Input: part model. Units: mm. Frame: model coordinates. A direction names the side the tool comes from. Coordinates: 2 decimals unless noted, no trailing zeros. Loops run counter-clockwise (first coordinate to the right, second up) from the corner with the lowest first, then second, coordinate; pieces in that order, holes last.
(1) Section A-A, the plane x = -22. Return loops of the section in (y, z).
(2) Section B-B, the plane y = 3. Return loops of the section in (x, z).
(3) Section C-C, the plane z = -48. Return loops of the section in (x, y).
(4) Section D-D, the plane z = 0. Return loops of the section in (x, y), then the cut area to 3 significant figures.
(5) Set-up query: faces 5 (the face through (-20, 24, -13)), 6 (the face through (6, 17, -1)), 7 (the face through (0, 15, -18)), 8 (the face through (17.44, 35.07, -33.96)), 9 (the face through (-13, 24, -8)). Return all of +Z, -Z, +X, -X, +Y, -Y with unobstructed straight access to the full face (end or side cutting, diameter ignored); none if empty.
(6) Mould query, pull axis X, two halves, no side actions, for faces 1 (the face through (1, 0, 0)), 2 (the face through (46, 4, 0)), 3 (the face through (35.932, 3.944, -1.041)), 4 (the face through (-6, 17, -1)). Classes: released by +X, released by -X, zero draft, split by the parting line, or undercut.
(7) Line query: L1, parallel to X at y = 6, z = 0; L2, parallel to Z at x = -15, y = 29.5; L3, parallel to Y at x = 5.5, z = -34. Output: solid intervals per line, ascending.
(8) Contact query for flat-ended pins moving along their axis: P1, Ø21, axis at x = -28, z = 0, coming from the +Y side; P2, Ø1, axis at x = -10.5, z = -39, coming from the -Y side; P3, Ø18, axis at x = 21, z = -7, coming from the +Y side. Output: stop coordinate, or through.
```python
from build123d import *

# Parameters (mm, degrees)
SKETCH2_R                = 8
BOSS_EXTRUDE1_DEPTH      = 8
SKETCH4_W                = 40
SKETCH4_H                = 10
BOSS_EXTRUDE2_DEPTH      = 32
BOSS_EXTRUDE3_DEPTH      = 6
BOSS_EXTRUDE3_DEPTH_BACK = 6
SKETCH7_R                = 10
BOSS_EXTRUDE4_DEPTH      = 10
BOSS_EXTRUDE5_START      = 10
SKETCH8_R                = 15
SKETCH8_R_2              = 10
BOSS_EXTRUDE5_DEPTH      = 10


with BuildPart() as part:
    # Sketch2 → Boss-Extrude1 (new body)
    with BuildSketch(Plane(origin=(0, 0, 0), x_dir=(1, 0, 0), z_dir=(0, 1, 0))):
        with BuildLine():
            Line((-28, 18), (28, 18))
            ThreePointArc((28, 18), (46, 0), (28, -18))
            Line((28, -18), (-28, -18))
            ThreePointArc((-28, -18), (-46, 0), (-28, 18))
        make_face()
        with Locations(Location((-28, 0, 0), (0, 0, 270))):
            Circle(SKETCH2_R, mode=Mode.SUBTRACT)
        with Locations(Location((28, 0, 0), (0, 0, 270))):
            Circle(SKETCH2_R, mode=Mode.SUBTRACT)
    extrude(amount=BOSS_EXTRUDE1_DEPTH)

    # Sketch4 → Boss-Extrude2 (add)
    with BuildSketch(Plane(origin=(0, 8, 0), x_dir=(1, 0, 0), z_dir=(0, 1, 0))):
        with Locations((0, 13)):
            Rectangle(SKETCH4_W, SKETCH4_H)
    extrude(amount=BOSS_EXTRUDE2_DEPTH)

    # Sketch5 → Boss-Extrude3 (add, two sides: drawn at the far end of the back side and taken through both)
    with BuildSketch(Plane(origin=(0, 0, 0), x_dir=(0, 0, -1), z_dir=(1, 0, 0)).offset(-BOSS_EXTRUDE3_DEPTH_BACK)):
        Polygon((8, 40), (8, 8), (-18, 8), align=None)
    extrude(amount=BOSS_EXTRUDE3_DEPTH + BOSS_EXTRUDE3_DEPTH_BACK)

    # Sketch7 → Boss-Extrude4 (add)
    with BuildSketch(Plane(origin=(0, 40, 0), x_dir=(1, 0, 0), z_dir=(0, 1, 0))):
        with BuildLine():
            Line((20, 18), (14.810951292, 50.373967528))
            ThreePointArc((14.810951292, 50.373967528), (0, 63), (-14.810951292, 50.373967528))
            Line((-14.810951292, 50.373967528), (-20, 18))
            Line((-20, 18), (20, 18))
        make_face()
        with Locations(Location((0, 48, 0), (0, 0, 270))):
            Circle(SKETCH7_R, mode=Mode.SUBTRACT)
    extrude(amount=-BOSS_EXTRUDE4_DEPTH)

    # Sketch8 → Boss-Extrude5 (add)
    with BuildSketch(Plane(origin=(0, 40, 0), x_dir=(1, 0, 0), z_dir=(0, 1, 0)).offset(BOSS_EXTRUDE5_START)):
        with Locations(Location((0, 48, 0), (0, 0, 270))):
            Circle(SKETCH8_R)
        with Locations(Location((0, 48, 0), (0, 0, 270))):
            Circle(SKETCH8_R_2, mode=Mode.SUBTRACT)
    extrude(amount=-BOSS_EXTRUDE5_DEPTH)


solid = part.part
```
Report:
1. outline: (0, -18) - (8, -18) - (8, -5.29) - (0, -5.29) - close; (0, 5.29) - (8, 5.29) - (8, 18) - (0, 18) - close
2. outline: (-28, -18) - (28, -18) arc R18 ccw to (28, 18) - (-28, 18) arc R18 ccw to start; hole circle Ø16 at (-28, 0); hole circle Ø16 at (28, 0)
3. outline: (-15.19, 30) - (-10, 30) - (-10, 50) - (-15, 50) - (-15, 40) - (-15.19, 40) - close; (10, 30) - (15.19, 30) - (15.19, 40) - (15, 40) - (15, 50) - (10, 50) - close
4. outline: (-46, 0) - (-36, 0) - (-36, 8) - (-46, 8) - close; (-20, 0) - (20, 0) - (20, 8) - (6, 8) - (6, 30.15) - (-6, 30.15) - (-6, 8) - (-20, 8) - close; (36, 0) - (46, 0) - (46, 8) - (36, 8) - close
4. area: 746 mm2
5. face 5: +Z, -Z, -X, +Y
5. face 6: +Z, +X, +Y
5. face 7: -Z, +X, -X, -Y
5. face 8: -Z, +X, +Y, -Y
5. face 9: +Z, -X, +Y
6. face 1: zero draft
6. face 2: released by +X
6. face 3: undercut
6. face 4: released by -X
7. L1: x = -46 to -36, -20 to 20, 36 to 46
7. L2: z = -18 to -8
7. L3: y = 30 to 40
8. P1: stops at y = 8
8. P2: stops at y = 30
8. P3: stops at y = 40
